Could you check a few things on this drawing? It's one solid part, dimensions in mm from its lowest x, y, z. Coordinates: 2 decimals unless noted, no trailing zeros. Order: outer loops, then holes, each group sorted by start corner. A loop starts at its lowest first (then second) coordinate and runs counter-clockwise, first axis right, second up. Notation, with made-up numbers: M 86,55.5 L 97,55.5 A10 ccw 97,68.5 Z; hole C 29,7.5 d10. An arc over 180 degrees is marked long. Answer as CSV lines item,"result". Start each with the question number.
1. I need wall thicknesses on line 1 along Z through (x, y) = (97, 10.5); line 2 along X through (y, z) = (6.5, 445). Which ranges of each line are inside material? Lowest first, please. Write a range as from..to.
2. If we section it at A-A (x = 34.5): List the corners of the cut face in (y, z) for me, plus the area to 3 significant figures.
3. If we section it at C-C (z = 375.5): List the corners of the cut face in (x, y) for me, plus the area to 3 significant figures.
4. If we section it at B-B (y = 8.25): List the corners of the cut face in (x, z) for me.
5. Will these pins go through, and if not, where does the flat tip stop? pin 1 (8 mm diameter, centred on y = 15.5, z = 375.5, fed in from +X); pin 2 (4 mm diameter, centred on y = 15, z = 488.5, fed in from -X).
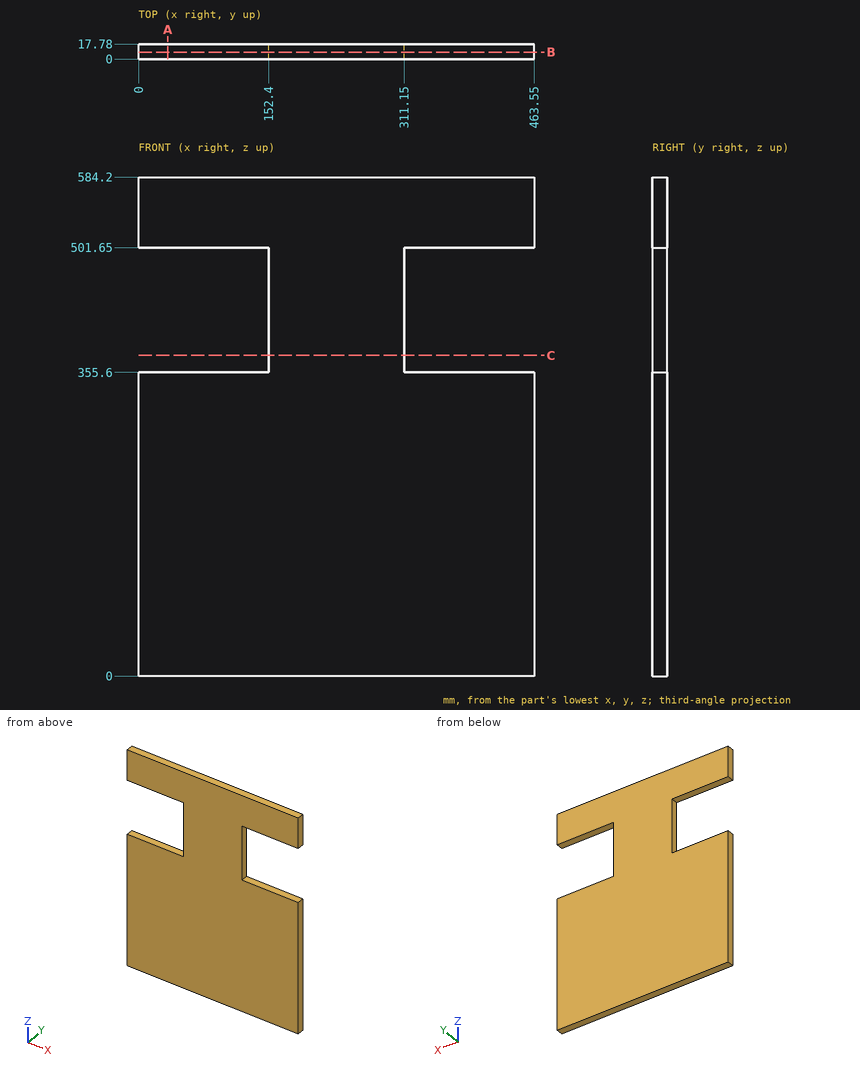
Solved:
1,line 1,"0..355.6, 501.65..584.2"
1,line 2,"152.4..311.15"
2,outline,"M 0,0 L 17.78,0 L 17.78,355.6 L 0,355.6 Z; M 0,501.65 L 17.78,501.65 L 17.78,584.2 L 0,584.2 Z"
2,area,"7,790 mm²"
3,outline,"M 152.4,0 L 311.15,0 L 311.15,17.78 L 152.4,17.78 Z"
3,area,"2,820 mm²"
4,outline,"M 0,0 L 463.55,0 L 463.55,355.6 L 311.15,355.6 L 311.15,501.65 L 463.55,501.65 L 463.55,584.2 L 0,584.2 L 0,501.65 L 152.4,501.65 L 152.4,355.6 L 0,355.6 Z"
5,pin 1,"x = 311.15"
5,pin 2,"x = 152.4"
